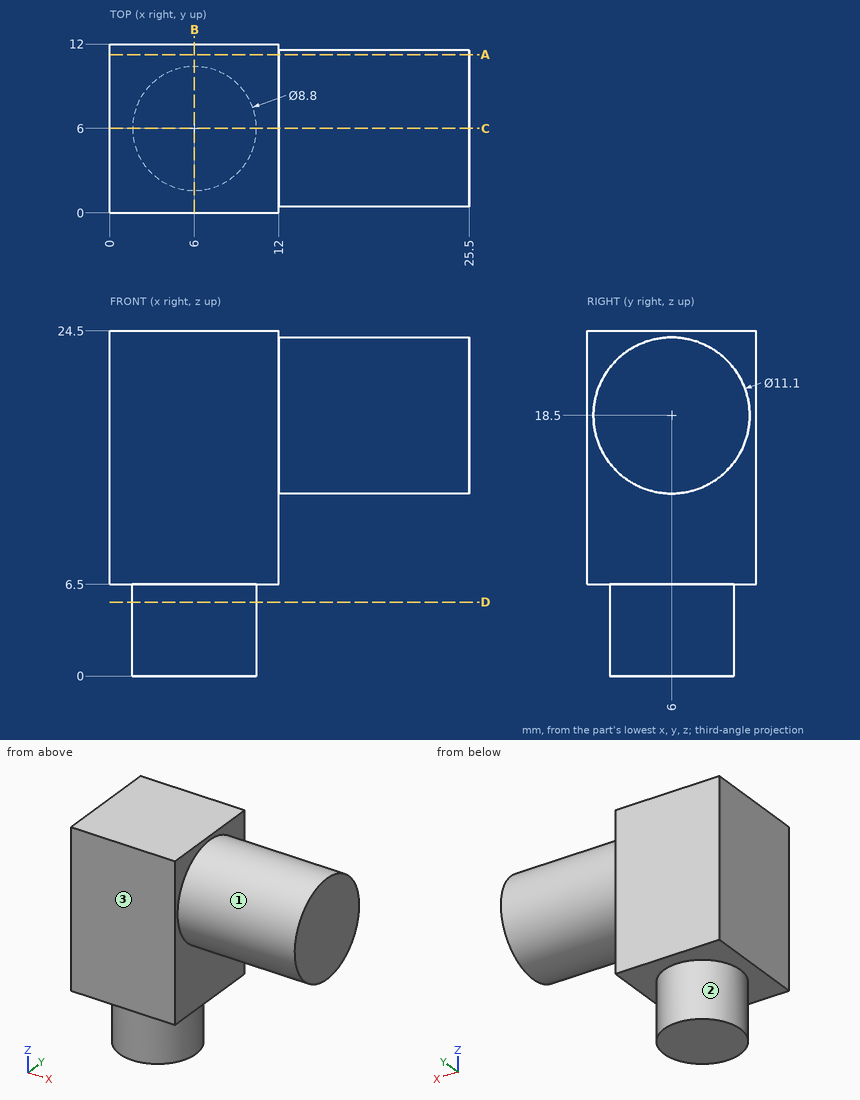
Study the drawing (mm; zero at the part's minimum x, y, z) and answer. A direction names the side the tool comes from. Coordinates: 2 decimals unless noted, no trailing zeros. Loops run counter-clockwise (first coordinate to the right, second up) from the corner with the lowest first, then second, coordinate; pieces in that order, holes last. Notation, with made-up numbers: (5.5, 17.25) -> (62.5, 17.25) arc R30 ccw to (62.5, 55.25) -> close; hole circle Ø8 at (31, 2). An arc over 180 degrees is marked (long way). Answer in a Markdown table with one row per item. Add a question column.
1. For the marked faces 1, 2 and 3, determine the directions among +Z, -Z, +X, -X, +Y, -Y from which every point of the face is accessible in a straight line to the end or side of a thin tool.
2. The part is cut by section B-B, the plane x = 6. Write down the section's boundary in (y, z), then the cut area to 3 significant figures.
3. The part is cut by section C-C, the plane y = 6. Write down the section's boundary in (x, z), then the cut area to 3 significant figures.
4. The part is cut by section D-D, the plane z = 5.25. Write down the section's boundary in (x, y), then the cut area to 3 significant figures.
5. Consider line 1 (X direction, y = 1, z = 14.25); line 2 (Z direction, x = 9, y = 2.75); line 3 (Z direction, x = 23.5, y = 10.25). Determine where each line is inside the solid, lowest interval first. Write a range as [from, to].
6. Flat-ended cylindrical pins translate along their axes: P1, Ø3.5, axis at y = 3.5, z = 13.5, coming from the +X side; P2, Ø6, axis at x = 20.5, y = 4, coming from the +Z side. Find the tip coordinate at first contact, or state that the pin passes through.
7. The part is cut by section A-A, the plane y = 11.25. Write down the section's boundary in (x, z).
Answer below:
| question | item | result |
|---|---|---|
| 1 | face 1 | +X |
| 1 | face 2 | -Z |
| 1 | face 3 | +Z, -Z, +X, -X, -Y |
| 2 | outline | (0, 6.5) -> (1.6, 6.5) -> (1.6, 0) -> (10.4, 0) -> (10.4, 6.5) -> (12, 6.5) -> (12, 24.5) -> (0, 24.5) -> close |
| 2 | area | 273 mm2 |
| 3 | outline | (0, 6.5) -> (1.6, 6.5) -> (1.6, 0) -> (10.4, 0) -> (10.4, 6.5) -> (12, 6.5) -> (12, 12.95) -> (25.5, 12.95) -> (25.5, 24.05) -> (12, 24.05) -> (12, 24.5) -> (0, 24.5) -> close |
| 3 | area | 423 mm2 |
| 4 | outline | circle Ø8.8 at (6, 6) |
| 4 | area | 60.8 mm2 |
| 5 | line 1 | [0, 12] |
| 5 | line 2 | [6.5, 24.5] |
| 5 | line 3 | [14.93, 22.07] |
| 6 | P1 | x = 25.5 |
| 6 | P2 | z = 24.05 |
| 7 | outline | (0, 6.5) -> (12, 6.5) -> (12, 16.7) -> (25.5, 16.7) -> (25.5, 20.3) -> (12, 20.3) -> (12, 24.5) -> (0, 24.5) -> close |
